Geometry: final body of the model. Coordinates: model frame, mm. Face numbers are marked on the shaded views. Give positions to 0.01 mm unless a question says otherwise; leave off trailing zeros. Loops run counter-clockwise (first coordinate to the right, second up) from the corner with the lowest first, then second, coordinate; pieces in that order, holes last.
1. Section D-D, the plane y = -20.75. Output: boundary loops of the cut face in (x, z).
2. Material intervals for line 1 along Y through (x, z) = (1.65, -4); line 2 along Y through (x, z) = (1.8, -5); line 3 along Z through (x, y) = (1.75, -20.75), sorted ascending.
3. Section A-A, the plane x = 1.3. State how many separate pieces and enclosed holes the cut face has, then the cut area to 3 significant figures.
4. Section C-C, the plane z = -1.75. Output: boundary loops of the cut face in (x, y), then the cut area to 3 significant figures.
5. Draft query along Y for the marked faces 1, 2, 3 and 4. Return one class per face: +Y half, -Y half, draft (parallel to the pull), parting line (faces both ways), or undercut.
6. First-contact query: P1, Ø2, axis at x = 0.5, y = -3, coming from the +Z side. Flat tip, straight axial feed; report the tip coordinate or a pass-through.
7. Section B-B, the plane z = -3.5. Output: boundary loops of the cut face in (x, y).
from build123d import *

# Parameters (mm, degrees)
SKETCH1_W           = 8
SKETCH1_H           = 27
BOSS_EXTRUDE1_DEPTH = 4
SKETCH2_R           = 2.5
SKETCH2_R_2         = 1.6
CUT_EXTRUDE1_DEPTH  = 29.442925307
FILLET1_R           = 4


with BuildPart() as part:
    # Sketch1 → Boss-Extrude1 (new body)
    with BuildSketch(Plane(origin=(0, 0, 0), x_dir=(0, 0, -1), z_dir=(1, 0, 0))):
        with Locations((4, -13.5)):
            Rectangle(SKETCH1_W, SKETCH1_H)
    extrude(amount=BOSS_EXTRUDE1_DEPTH)

    # Sketch2 → Cut-Extrude1 (cut, through all)
    with BuildSketch(Plane(origin=(4, 0, 0), x_dir=(0, 0, -1), z_dir=(1, 0, 0))):
        with Locations((4, -23)):
            Circle(SKETCH2_R)
        with Locations((4, -4)):
            Circle(SKETCH2_R_2)
    extrude(amount=-CUT_EXTRUDE1_DEPTH, mode=Mode.SUBTRACT)

    # Fillet1
    fillet1_edges = [part.edges().sort_by_distance(p)[0] for p in [
        (2, -27, -8),
        (2, -27, 0),
        (2, 0, 0),
        (2, 0, -8),
    ]]
    fillet(fillet1_edges, radius=FILLET1_R - 0.0001)  # a hair under: the kernel refuses the full size


solid = part.part
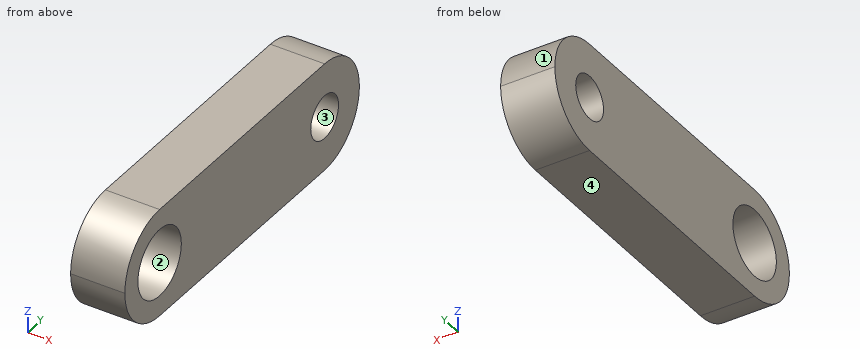
Answers below:
1. outline: (0, -8) - (4, -8) - (4, -5.09) - (0, -5.09) - close; (0, -2.91) - (4, -2.91) - (4, 0) - (0, 0) - close
2. line 1: y = -27 to -25.5, -20.5 to -5.6, -2.4 to 0
2. line 2: y = -26.87 to -25.29, -20.71 to -5.25, -2.75 to -0.13
2. line 3: z = -8 to -5.09, -2.91 to 0
3. separate pieces: 1
3. enclosed holes: 2
3. area: 175 mm2
4. outline: (0, -26.31) - (4, -26.31) - (4, -24.09) - (0, -24.09) - close; (0, -21.91) - (4, -21.91) - (4, -0.69) - (0, -0.69) - close
4. area: 93.7 mm2
5. face 1: +Y half
5. face 2: undercut
5. face 3: undercut
5. face 4: draft
6. P1: stops at z = 0
7. outline: (0, -26.97) - (4, -26.97) - (4, -25.45) - (0, -25.45) - close; (0, -20.55) - (4, -20.55) - (4, -5.52) - (0, -5.52) - close; (0, -2.48) - (4, -2.48) - (4, -0.03) - (0, -0.03) - close
